Verification items for the finished model (mm, model axes). Coordinates: 2 decimals unless noted, no trailing zeros. Order: outer loops, then holes, each group sorted by start corner. A loop starts at its lowest first (then second) coordinate and runs counter-clockwise, first axis right, second up. Notation, with made-up numbers: (-17, -22) -> (17, -22) arc R15 cw to (17, -7) -> close; hole circle Ø8 at (-22.5, -30.75). An arc over 180 degrees is marked (long way). Answer as CSV lines item,"result".
```python
from build123d import *

# Parameters (mm, degrees)
F0_R          = 5.08
F0_R_2        = 1.19126
F1_DEPTH      = 3.175
F2_SIZE       = 0.127
F3_R          = 0.79375
F4_DEPTH      = 25.4
F4_DEPTH_BACK = 25.4


with BuildPart() as f1:
    # F0 (on Front) → F1 (new body)
    with BuildSketch(Plane.XZ):
        Circle(F0_R)
        Circle(F0_R_2, mode=Mode.SUBTRACT)
    extrude(amount=F1_DEPTH)

    # F2
    f2_edges = [f1.edges().sort_by_distance(p)[0] for p in [
        (-5.08, -3.175, 0),
    ]]
    chamfer(f2_edges, length=F2_SIZE)

    # F3 (on Front) → F4 (cut, two sides)
    with BuildSketch(Plane.XZ) as f4_sk:
        with Locations((-2.794, 0)):
            Circle(F3_R)
    extrude(amount=-F4_DEPTH, mode=Mode.SUBTRACT)
    extrude(f4_sk.sketch, amount=F4_DEPTH_BACK, mode=Mode.SUBTRACT)


solid = f1.part
```
Item 1: Section check B-B, the plane z = 0. Record the boundary of the cut face in (x, y) (3 decimals).
Answer list:
outline,"(-5.08, -3.048) -> (-4.953, -3.175) -> (-3.588, -3.175) -> (-3.588, 0) -> (-5.08, 0) -> close; (-2, -3.175) -> (-1.191, -3.175) -> (-1.191, 0) -> (-2, 0) -> close; (1.191, -3.175) -> (4.953, -3.175) -> (5.08, -3.048) -> (5.08, 0) -> (1.191, 0) -> close"
Item 2: Thickness scan on line 1 (Z direction, x = 0, y = -2.85); line 2 (X direction, y = -1.8, z = -0.5); line 3 (X direction, y = -0.7, z = 0.25). Record the ranges inside material, lowest first.
Answer list:
line 1,"-5.08 to -1.19, 1.19 to 5.08"
line 2,"-5.06 to -3.41, -2.18 to -1.08, 1.08 to 5.06"
line 3,"-5.07 to -3.55, -2.04 to -1.16, 1.16 to 5.07"
Item 3: Depth check by flat-ended pin: pin 1 Ø1 at (x, z) = (-2.794, 0) entering from +Y. Enter the tip coordinate at first touch or a pass-through.
Answer list:
pin 1,"through"
Item 4: Section check C-C, the plane y = -0.85. Record the boundary of the cut face in (x, z).
Answer list:
outline,"circle Ø10.16 at (0, 0); hole circle Ø1.59 at (-2.79, 0); hole circle Ø2.38 at (0, 0)"
Item 5: Release check for a two-part mould opening along Z. For faces 1 (the flat face through (1, -3.175, -1)), 2 (the cylindrical face through (-2, -2, 0)), 3 (the cylindrical face through (-0.661, -1.503, 5.037)) record: +Z half, -Z half, draft (parallel to the pull), parting line (faces both ways), or undercut.
Answer list:
face 1,"draft"
face 2,"undercut"
face 3,"parting line"
Item 6: Section check A-A, the plane x = 0. Record the boundary of the cut face in (y, z) (3 decimals), plus the area to 3 significant figures.
Answer list:
outline,"(-3.175, -4.953) -> (-3.048, -5.08) -> (0, -5.08) -> (0, -1.191) -> (-3.175, -1.191) -> close; (-3.175, 1.191) -> (0, 1.191) -> (0, 5.08) -> (-3.048, 5.08) -> (-3.175, 4.953) -> close"
area,"24.7 mm2"
